Can you work these out from the model? Positions are in its coordinate system, mm. Face numbers are marked on the shaded views. A direction names the side the tool comes from. Coordinates: 2 decimals unless noted, no trailing zeros. Order: outer loops, then holes, each group sorted by start corner. A loop starts at its lowest first (then second) coordinate and runs counter-clockwise, first axis right, second up. Notation, with made-up numbers: (28, 21) -> (73, 21) arc R37 ccw to (73, 59) -> close; hole circle Ø7 at (48, -13). An arc over 180 degrees is marked (long way). Answer as CSV lines item,"result".
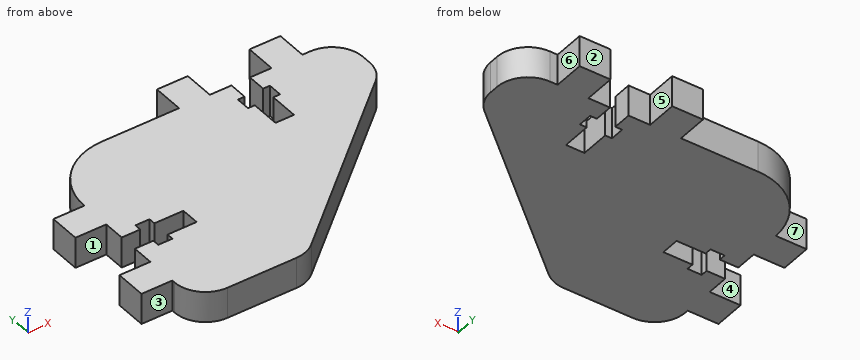
from build123d import *

# Parameters (mm, degrees)
BOSS_EXTRUDE1_DEPTH = 5
FILLET1_R           = 10
FILLET2_R           = 5


with BuildPart() as part:
    # Sketch1 → Boss-Extrude1 (new body)
    with BuildSketch(Plane.XY):
        Polygon((-92.5, 96.5), (-92.5, 100), (-97.5, 100), (-97.5, 105), (-92.5, 105), (-92.5, 115), (-70, 115), (-70, 120), (-65, 120), (-65, 115), (-61.5, 115), (-61.5, 112), (-62.6, 112), (-62.6, 109.7), (-61.5, 109.7), (-61.5, 105), (-58.5, 105), (-58.5, 109.7), (-57.4, 109.7), (-57.4, 112), (-58.5, 112), (-58.5, 115), (-55, 115), (-55, 120), (-50, 120), (-50, 115), (-43.75587644, 115), (-43.75587644, 106.227080611), (-74.442868217, 79.497668649), (-92.5, 79.497668649), (-92.5, 85), (-97.5, 85), (-97.5, 90), (-92.5, 90), (-92.5, 93.5), (-89.5, 93.5), (-89.5, 92.4), (-87.2, 92.4), (-87.2, 93.5), (-82.5, 93.5), (-82.5, 96.5), (-87.2, 96.5), (-87.2, 97.6), (-89.5, 97.6), (-89.5, 96.5), align=None)
    extrude(amount=BOSS_EXTRUDE1_DEPTH)

    # Fillet1
    fillet1_edges = [part.edges().sort_by_distance(p)[0] for p in [
        (-92.5, 115, 2.5),
    ]]
    fillet(fillet1_edges, radius=FILLET1_R - 0.0001)  # a hair under: the kernel refuses the full size

    # Fillet2
    fillet2_edges = [part.edges().sort_by_distance(p)[0] for p in [
        (-43.75587644, 115, 2.5),
        (-43.75587644, 106.227080611, 2.5),
        (-74.442868217, 79.497668649, 2.5),
        (-92.5, 79.497668649, 2.5),
    ]]
    fillet(fillet2_edges, radius=FILLET2_R)


solid = part.part
Q1. Imagine slicing it at B-B (y = 91.5). List the corners of the cut face in (x, z) for me.
Solution:
outline,"(-92.5, 0) -> (-60.66, 0) -> (-60.66, 5) -> (-92.5, 5) -> close"
Q2. We'd pull the mould along Y, two halves only. Please class the marked faces 1, 2 and 3: pulls with the +Y half, pulls with the -Y half, needs draft (parallel to the pull), parting line crosses it, or undercut.
Solution:
face 1,"undercut"
face 2,"pulls with the +Y half"
face 3,"pulls with the -Y half"
Q3. Which directions (+Z, -Z, +X, -X, +Y, -Y) give clear straight access to the entire face, cutting with the end or side of a thin tool? Please do the marked faces 4, 5, 6 and 7.
Solution:
face 4,"+Z, -Z, -X"
face 5,"+Z, -Z, +Y"
face 6,"+Z, -Z, +X, +Y"
face 7,"+Z, -Z, -X, +Y"
Q4. Imagine slicing it at A-A (x = -77.5). List the corners of the cut face in (y, z) for me.
Solution:
outline,"(79.5, 0) -> (115, 0) -> (115, 5) -> (79.5, 5) -> close"
Q5. For P1, Ø1.5, axis at x = -62.5, y = 97.5, coming from the -Z side; P2, Ø3, axis at x = -69, z = 2, coming from the -Y side; P3, Ø2.5, axis at y = 117, z = 1.5, coming from the +X side; P4, Ø0.9, axis at y = 95.5, z = 3.5, coming from the -X side, each with a flat end and sliding along its axis, tell me the tip position at first contact or that it passes through.
Solution:
P1,"z = 0"
P2,"y = 82.93"
P3,"x = -50"
P4,"x = -82.5"
Q6. If I drill on line 1 (Y direction, x = -95, z = 4.3); line 2 (X direction, y = 92.5, z = 4.7); line 3 (X direction, y = 117, z = 2.3), over which ranges is the centre line in solid material (lowest first)?
Solution:
line 1,"85 to 90, 100 to 105"
line 2,"-92.5 to -89.5, -87.2 to -59.52"
line 3,"-70 to -65, -55 to -50"
